For this review, take the finished solid that the model builds, in its own axes (mm). Round coordinates to 2 decimals unless told otherwise and drop trailing zeros. Order: outer loops, then holes, each group sorted by start corner. A loop starts at its lowest first (then second) coordinate and runs counter-clockwise, first axis right, second up. Notation, with made-up numbers: M -31.5,-16.5 L -5.5,-16.5 A20 ccw -5.5,-10.5 Z; hole C 77.5,5.25 d1. An arc over 180 degrees is marked long. Put each result on its own line as item: value.
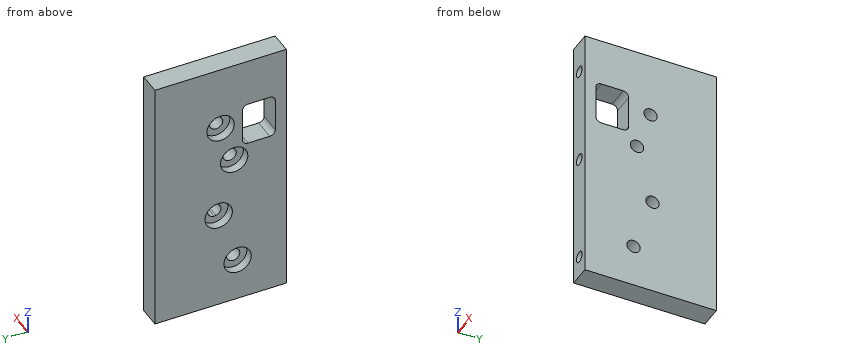
from build123d import *

# Parameters (mm, degrees)
SKETCH1_R                       = 3.854557775
BOSS_EXTRUDE1_DEPTH             = 12.7
F_1_4_0_25_DIAMETER_HOLE2_D     = 6.35
F_1_4_0_25_DIAMETER_HOLE2_DEPTH = 38.1
F_1_4_0_25_DIAMETER_HOLE2_TIP   = 1.907732465
SKETCH2_R                       = 7.9375
CUT_EXTRUDE1_DEPTH              = 5.08
CUT_EXTRUDE2_DEPTH              = 87.135590786


with BuildPart() as part:
    # Sketch1 → Boss-Extrude1 (new body)
    # profile 1 of 2: a face of its own
    with BuildSketch(Plane(origin=(0, 0, 0), x_dir=(0, 0, -1), z_dir=(1, 0, 0))):
        with BuildLine():
            Line((-76.2, 38.1), (-76.2, 0))
            Line((-76.2, 0), (-41.954557775, 0))
            ThreePointArc((-41.954557775, 0), (-38.1, 3.854557775), (-34.245442225, 0))
            Line((-34.245442225, 0), (14.762299925, 0))
            ThreePointArc((14.762299925, 0), (17.903949731, 4.910646748), (22.312291357, 1.096077429))
            ThreePointArc((22.312291357, 1.096077429), (22.272302901, 0.542293578), (22.153167239, 0))
            Line((22.153167239, 0), (76.2, 0))
            Line((76.2, 0), (76.2, 38.1))
            Line((76.2, 38.1), (-76.2, 38.1))
        make_face()
    # profile 2 of 2: a face of its own
    with BuildSketch(Plane(origin=(0, 0, 0), x_dir=(0, 0, -1), z_dir=(1, 0, 0))):
        with BuildLine():
            Line((-41.954557775, 0), (-76.2, 0))
            Line((-76.2, 0), (-76.2, -38.1))
            Line((-76.2, -38.1), (76.2, -38.1))
            Line((76.2, -38.1), (76.2, 0))
            Line((76.2, 0), (22.153167239, 0))
            ThreePointArc((22.153167239, 0), (18.457733582, -2.758480346), (14.762299925, 0))
            Line((14.762299925, 0), (-34.245442225, 0))
            ThreePointArc((-34.245442225, 0), (-38.1, -3.854557775), (-41.954557775, 0))
        make_face()
        with Locations((-14.836022013, -7.860160654)):
            Circle(SKETCH1_R, mode=Mode.SUBTRACT)
        with Locations((51.143457994, -9.873506971)):
            Circle(SKETCH1_R, mode=Mode.SUBTRACT)
    extrude(amount=BOSS_EXTRUDE1_DEPTH)

    # 1_4 _0.25_ Diameter Hole2
    with Locations(Plane.XZ.offset(38.1)):
        with Locations((6.35, 57.15), (6.35, -63.5), (6.35, 0)):
            Hole(F_1_4_0_25_DIAMETER_HOLE2_D / 2, depth=F_1_4_0_25_DIAMETER_HOLE2_DEPTH)
            with Locations((0, 0, -(F_1_4_0_25_DIAMETER_HOLE2_DEPTH + F_1_4_0_25_DIAMETER_HOLE2_TIP / 2))):  # 118° drill point
                Cone(0, F_1_4_0_25_DIAMETER_HOLE2_D / 2, F_1_4_0_25_DIAMETER_HOLE2_TIP, mode=Mode.SUBTRACT)

    # Sketch2 → Cut-Extrude1 (cut)
    with BuildSketch(Plane.ZY):
        with Locations((38.1, 0)):
            Circle(SKETCH2_R)
        with Locations((14.836022013, -7.860160654)):
            Circle(SKETCH2_R)
        with Locations((-18.457733582, 1.096077429)):
            Circle(SKETCH2_R)
        with Locations((-51.143457994, -9.873506971)):
            Circle(SKETCH2_R)
    extrude(amount=-CUT_EXTRUDE1_DEPTH, mode=Mode.SUBTRACT)

    # Sketch5 → Cut-Extrude2 (cut, through all)
    with BuildSketch(Plane.ZY):
        with BuildLine():
            Line((26.035, -12.7), (45.085, -12.7))
            ThreePointArc((45.085, -12.7), (47.33006403, -13.62993597), (48.26, -15.875))
            Line((48.26, -15.875), (48.26, -28.575))
            ThreePointArc((48.26, -28.575), (47.33006403, -30.82006403), (45.085, -31.75))
            Line((45.085, -31.75), (26.035, -31.75))
            ThreePointArc((26.035, -31.75), (23.78993597, -30.82006403), (22.86, -28.575))
            Line((22.86, -28.575), (22.86, -15.875))
            ThreePointArc((22.86, -15.875), (23.78993597, -13.62993597), (26.035, -12.7))
        make_face()
    extrude(amount=-CUT_EXTRUDE2_DEPTH, mode=Mode.SUBTRACT)


solid = part.part
(1) Add section B-B on z = 38.1. Give the boundary of the cut face in (x, y), then the cut area to 3 significant figures.
A:
outline: M 0,-38.1 L 12.7,-38.1 L 12.7,-31.75 L 0,-31.75 Z; M 0,-12.7 L 12.7,-12.7 L 12.7,-3.85 L 5.08,-3.85 L 5.08,-7.94 L 0,-7.94 Z; M 0,7.94 L 5.08,7.94 L 5.08,3.85 L 12.7,3.85 L 12.7,38.1 L 0,38.1 Z
area: 586 mm2
(2) Add section C-C on x = 11. State how many separate pieces and enclosed holes the cut face has, then the cut area to 3 significant figures.
A:
separate pieces: 1
enclosed holes: 5
area: 11,000 mm2
(3) To check wall thickness, follow L1, parallel to Y at x = 11, z = 38.1; L2, parallel to Y at x = 2, z = 44.5; L3, parallel to Z at x = 1, y = -16. State the ranges of each line that lie inside material, in increasing order.
A:
L1: y = -38.1 to -31.75, -12.7 to -3.85, 3.85 to 38.1
L2: y = -38.1 to -31.75, -12.7 to -4.7, 4.7 to 38.1
L3: z = -76.2 to -56.19, -46.1 to 22.86, 48.26 to 76.2
(4) Add section A-A on y = -21. Give the boundary of the cut face in (x, z) (3 decimals), then the cut area to 3 significant figures.
A:
outline: M 0,-76.2 L 12.7,-76.2 L 12.7,22.86 L 0,22.86 Z; M 0,48.26 L 12.7,48.26 L 12.7,76.2 L 0,76.2 Z; hole C 6.35,-63.5 d6.35; hole C 6.35,0 d6.35; hole C 6.35,57.15 d6.35
area: 1,520 mm2
(5) Insertion check: pin 1 Ø1 at (y, z) = (-23.5, 12) entering from -X; pin 2 Ø8 at (y, z) = (3.5, -20.5) entering from -X; pin 3 Ø5.5 at (x, z) = (6.35, -63.5) entering from -Y. Each pin has a flat end and moves straight along its axis. Give the tip position at first contact, or say it passes through.
A:
pin 1: stops at x = 0
pin 2: stops at x = 5.08
pin 3: stops at y = 0.26
